Drawing for the job (mm, zero at the part's lowest x, y, z). A direction names the side the tool comes from. Round coordinates to 2 decimals unless told otherwise and drop trailing zeros. Order: outer loops, then holes, each group sorted by start corner. A loop starts at its lowest first (then second) coordinate and runs counter-clockwise, first axis right, second up. Notation, with made-up numbers: (73, 50.5) -> (130, 50.5) arc R21 ccw to (130, 82.5) -> close; hole circle Ø7 at (54, 68). An arc over 180 degrees is marked (long way). Use CSV: the item, a comma, the result in double quotes.
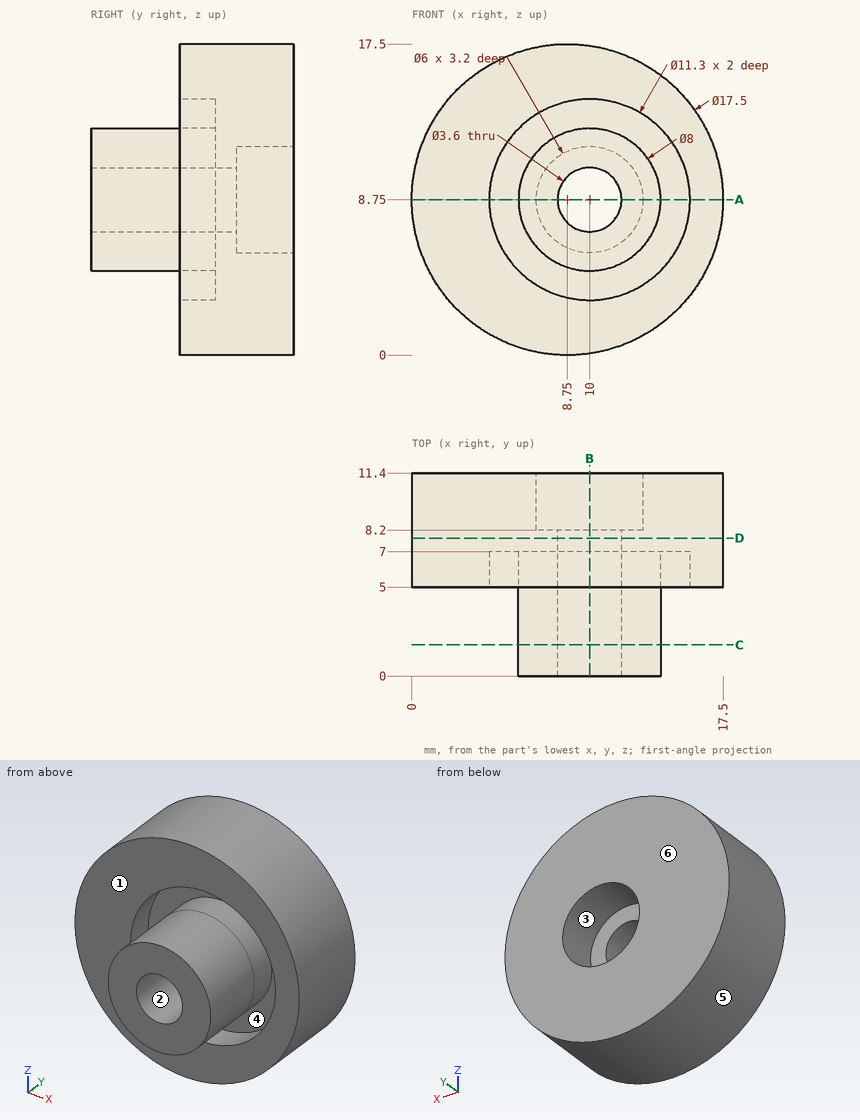
Q1. Cut at A-A (z = 8.75). Give the cut face in (x, y).
From the geometry:
outline,"(0, 5) -> (4.35, 5) -> (4.35, 7) -> (6, 7) -> (6, 0) -> (8.2, 0) -> (8.2, 8.2) -> (7, 8.2) -> (7, 11.4) -> (0, 11.4) -> close; (11.8, 0) -> (14, 0) -> (14, 7) -> (15.65, 7) -> (15.65, 5) -> (17.5, 5) -> (17.5, 11.4) -> (13, 11.4) -> (13, 8.2) -> (11.8, 8.2) -> close"
Q2. Cut at D-D (y = 7.75). Give the cut face in (x, z).
From the geometry:
outline,"circle Ø17.5 at (8.75, 8.75); hole circle Ø3.6 at (10, 8.75)"
Q3. Pin check, flat tips, straight feed: pin 1 (6 mm diameter, centred on x = 2.5, z = 4.5, fed in from -Y); pin 2 (1 mm diameter, centred on x = 10, y = 10, fed in from -Z); pin 3 (2 mm diameter, centred on x = 10, z = 8.75, fed in from -Y); pin 4 (2 mm diameter, centred on y = 8, z = 12, fed in from -X). Stop position of each tip, or through.
From the geometry:
pin 1,"stops at y = 5"
pin 2,"stops at z = 0.03"
pin 3,"passes through"
pin 4,"stops at x = 0.29"
Q4. Cut at B-B (x = 10). Give the cut face in (y, z), plus the area to 3 significant figures.
From the geometry:
outline,"(0, 4.75) -> (7, 4.75) -> (7, 3.1) -> (5, 3.1) -> (5, 0.09) -> (11.4, 0.09) -> (11.4, 5.75) -> (8.2, 5.75) -> (8.2, 6.95) -> (0, 6.95) -> close; (0, 10.55) -> (8.2, 10.55) -> (8.2, 11.75) -> (11.4, 11.75) -> (11.4, 17.41) -> (5, 17.41) -> (5, 14.4) -> (7, 14.4) -> (7, 12.75) -> (0, 12.75) -> close"
area,"95.5 mm²"
Q5. Cut at C-C (y = 1.75). Give the cut face in (x, z).
From the geometry:
outline,"circle Ø8 at (10, 8.75); hole circle Ø3.6 at (10, 8.75)"
Q6. Which spindle directions (+Z, -Z, +X, -X, +Y, -Y) get a long thin tool onto all of the face, cutting with end or side? Do the marked faces 1, 2 and 3. Say none if no direction does.
From the geometry:
face 1,"-Y"
face 2,"+Y, -Y"
face 3,"+Y"
Q7. Mould opens along X. For the marked faces 4, 5 and 6 say: +X half, -X half, draft (parallel to the pull), parting line (faces both ways), or undercut.
From the geometry:
face 4,"undercut"
face 5,"parting line"
face 6,"draft"
Q8. Probe line 1 along X through (y, z) = (10.15, 8.75); line 2 along Z through (x, y) = (10, 5.75); line 3 along Y through (x, z) = (5.5, 7.75). List the from-to ranges inside material, lowest first.
From the geometry:
line 1,"x = 0 to 7, 13 to 17.5"
line 2,"z = 0.09 to 3.1, 4.75 to 6.95, 10.55 to 12.75, 14.4 to 17.41"
line 3,"y = 7 to 11.4"
